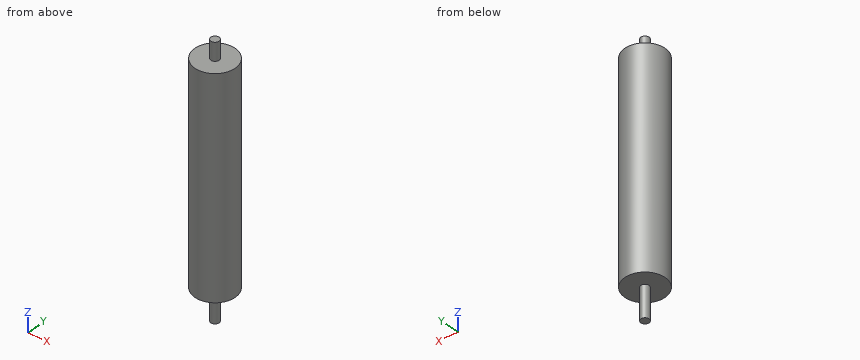
Autodesk Inventor part; units mm, degrees
ref_plane "YZ Plane" through (0, 0, 0) normal (1, 0, 0) x (0, 1, 0)
ref_plane "XZ Plane" through (0, 0, 0) normal (0, 1, 0) x (-1, 0, 0)
ref_plane "XY Plane" through (0, 0, 0) normal (0, 0, 1) x (1, 0, 0)
sketch "草图1" plane through (0, 0, 0) normal (0, 0, 1) x (1, 0, 0)
  circle A0 centre (0, 0) radius 4.6
  dimension "d0" = 9.2
extrude "拉伸1" add sketch "草图1" along normal blind 20
sketch "草图2" plane through (0, 0, 0) normal (0, 0, -1) x (-1, 0, 0)
  circle A0 centre (0, 0) radius 4.6
  circle A1 centre (0, 0) radius 22.5
  dimension "d3" = 45
extrude "拉伸2" add sketch "草图2" along normal blind 240 contours A0 | A1
sketch "草图3" plane through (0, 0, -240) normal (0, 0, -1) x (-1, 0, 0)
  circle A0 centre (0, 0) radius 4.6
  circle A1 centre (0, 0) radius 4.6
extrude "拉伸3" add sketch "草图3" along normal blind 35
properties part number "滚轴1"
Build history of the part. All positions in model axes, mm. Round coordinates to 2 decimals unless told otherwise and drop trailing zeros. Write each loop counter-clockwise with the first axis right and the second up, starting at its lowest first coordinate (ties: lowest second). Pieces come first, ordered by that corner, then holes. Notation, with made-up numbers: M 23.5,-37.75 L 28.5,-37.75 A11 ccw 28.5,-19.75 Z; hole C -26,19 d6. An arc over 180 degrees is marked long. Answer as a JSON object with one key per item and string values. Group by question number.
(1) Cut at A-A (x = 0). Give the cut face in (y, z).
(2) Cut at D-D (x = -19). Give the cut face in (y, z), and give its area (3 significant figures).
(3) Drill centre lines: L1, parallel to Z at x = 4, y = 18.5; L2, parallel to Y at x = -0.5, z = -42; L3, parallel to X at y = 4, z = -151. Where is each one in solid material? Low to high.
(4) Flat gauge pins, fed straight in: pin 1 (2 mm diameter, centred on x = 8, y = -17.5, fed in from -Z); pin 2 (5 mm diameter, centred on x = 5.5, z = -173.5, fed in from +Y); pin 3 (10 mm diameter, centred on x = -16, z = -74.5, fed in from -Y). Where does each tip first touch, or does it go through?
(5) Cut at C-C (z = -64). Give the cut face in (x, y).
Responses:
{
 "1": {"outline": "M -22.5,-240 L -4.6,-240 L -4.6,-275 L 4.6,-275 L 4.6,-240 L 22.5,-240 L 22.5,0 L 4.6,0 L 4.6,20 L -4.6,20 L -4.6,0 L -22.5,0 Z"},
 "2": {"outline": "M -12.05,-240 L 12.05,-240 L 12.05,0 L -12.05,0 Z", "area": "5,780 mm2"},
 "3": {"L1": "z = -240 to 0", "L2": "y = -22.49 to 22.49", "L3": "x = -22.14 to 22.14"},
 "4": {"pin 1": "stops at z = -240", "pin 2": "stops at y = 22.3", "pin 3": "stops at y = -19.63"},
 "5": {"outline": "C 0,0 d45"}
}
